from build123d import *

# Parameters (mm, degrees)
BOSS_EXTRUDE1_DEPTH = 2.8575
SKETCH3_R           = 2.55
CUT_EXTRUDE1_DEPTH  = 6.715
SKETCH4_R           = 2.55
CUT_EXTRUDE2_DEPTH  = 5.715


with BuildPart() as part:
    # Sketch2 → Boss-Extrude1 (new body, symmetric)
    with BuildSketch(Plane.XY):
        with BuildLine():
            Line((-20, 10), (20, 10))
            ThreePointArc((20, 10), (30, 0), (20, -10))
            Line((20, -10), (-20, -10))
            ThreePointArc((-20, -10), (-30, 0), (-20, 10))
        make_face()
    extrude(amount=BOSS_EXTRUDE1_DEPTH, both=True)

    # Sketch3 → Cut-Extrude1 (cut, through all)
    with BuildSketch(Plane.XY.offset(2.8575)):
        with Locations((9, 0)):
            Circle(SKETCH3_R)
        with Locations((23, 0)):
            Circle(SKETCH3_R)
    extrude(amount=-CUT_EXTRUDE1_DEPTH, mode=Mode.SUBTRACT)

    # Sketch4 → Cut-Extrude2 (cut)
    with BuildSketch(Plane.XY.offset(2.8575)):
        with Locations((-19.85, 0)):
            Circle(SKETCH4_R)
    extrude(amount=-CUT_EXTRUDE2_DEPTH, mode=Mode.SUBTRACT)


solid = part.part
CAD build for the part. Positions are in the model's coordinates, mm. Round coordinates to 2 decimals unless told otherwise and drop trailing zeros. Loops run counter-clockwise (first coordinate to the right, second up) from the corner with the lowest first, then second, coordinate; pieces in that order, holes last. Notation, with made-up numbers: (-7.75, 61) - (25.25, 61) arc R33 cw to (25.25, 100) - close; hole circle Ø5 at (83, -12.5). An arc over 180 degrees is marked (long way). Put each result on its own line as item: value.
1. Two-plate mould, pull along X, no slides. Class faces 1 (the cylindrical face through (20.452, 0.112, 0.04)), 2 (the cylindrical face through (-30, 0, 0)), 3 (the flat face through (0, 10, 0)): released by +X, released by -X, zero draft, split by the parting line, or undercut.
Geometry check:
face 1: undercut
face 2: released by -X
face 3: zero draft
2. Slice it at D-D on y = -6. List the corners of the cut face in (x, z), and give its area (3 significant figures).
Geometry check:
outline: (-28, -2.86) - (28, -2.86) - (28, 2.86) - (-28, 2.86) - close
area: 320 mm²
3. Slice it at B-B on y = 0. List the corners of the cut face in (x, z), and give its area (3 significant figures).
Geometry check:
outline: (-30, -2.86) - (-22.4, -2.86) - (-22.4, 2.86) - (-30, 2.86) - close; (-17.3, -2.86) - (6.45, -2.86) - (6.45, 2.86) - (-17.3, 2.86) - close; (11.55, -2.86) - (20.45, -2.86) - (20.45, 2.86) - (11.55, 2.86) - close; (25.55, -2.86) - (30, -2.86) - (30, 2.86) - (25.55, 2.86) - close
area: 255 mm²
4. Slice it at C-C on z = -0.35. List the corners of the cut face in (x, y), and give its area (3 significant figures).
Geometry check:
outline: (-20, -10) - (20, -10) arc R10 ccw to (20, 10) - (-20, 10) arc R10 ccw to start; hole circle Ø5.1 at (-19.85, 0); hole circle Ø5.1 at (9, 0); hole circle Ø5.1 at (23, 0)
area: 1,050 mm²
5. Slice it at A-A on x = 9. List the corners of the cut face in (y, z), and give its area (3 significant figures).
Geometry check:
outline: (-10, -2.86) - (-2.55, -2.86) - (-2.55, 2.86) - (-10, 2.86) - close; (2.55, -2.86) - (10, -2.86) - (10, 2.86) - (2.55, 2.86) - close
area: 85.2 mm²
6. Pin check, flat tips, straight feed: P1, Ø2, axis at y = -6.5, z = -2, coming from the +X side; P2, Ø4.5, axis at x = 9, y = 0, coming from the -Z side. Stop position of each tip, or through.
Geometry check:
P1: x = 28.35
P2: through
7. Wall check: line 1 (Y direction, x = -19.85, z = 0.65); line 2 (X direction, y = -0.75, z = 2.6); line 3 (Y direction, x = 23, z = 1.6). Give the ranges that are in metal, low to high.
Geometry check:
line 1: -10 to -2.55, 2.55 to 10
line 2: -29.97 to -22.29, -17.41 to 6.56, 11.44 to 20.56, 25.44 to 29.97
line 3: -9.54 to -2.55, 2.55 to 9.54
